Autodesk Fusion 360 part; units mm, degrees
sketch "Sketch1" plane through (0, 0, 0) normal (0, 0, 1) x (1, 0, 0)
  line L0 (0, 0) -> (84.5, 0)
  line L1 (84.5, 0) -> (84.5, 126.75)
  line L2 (84.5, 126.75) -> (0, 126.75)
  line L3 (0, 126.75) -> (0, 0)
  line L4 (0, 126.75) -> (5, 126.75)
  line L5 (5, 126.75) -> (5, 121.75)
  line L6 (5, 121.75) -> (0, 121.75)
  line L7 (0, 121.75) -> (0, 126.75)
  line L8 (84.5, 0) -> (79.5, 0)
  line L9 (79.5, 0) -> (79.5, 5)
  line L10 (79.5, 5) -> (84.5, 5)
  line L11 (84.5, 5) -> (84.5, 0)
  line L12 (5, 121.75) -> (79.5, 121.75)
  line L13 (79.5, 121.75) -> (79.5, 5)
  line L14 (79.5, 5) -> (5, 5)
  line L15 (5, 5) -> (5, 121.75)
  dimension "d1" = 84.5
  dimension "d2" = 126.75
  dimension "d3" = 5
  dimension "d4" = 5
  dimension "d5" = 5
  dimension "d6" = 5
extrude "Extrude1" add sketch "Sketch1" along normal blind 22 contours L0 L3 L6 L9 L14 L15 | L0 L1 L8 L9 L10 L11 | L2 L3 L4 L5 L6 L7 | L1 L2 L5 L10 L12 L13 makes body 1
sketch "Sketch2" plane through (0, 0, 22) normal (0, 0, 1) x (-1, 0, 0)
  line L0 (-79.5, -5) -> (-5, -5)
  line L1 (-5, -5) -> (-5, -121.75)
  line L2 (-5, -121.75) -> (-79.5, -121.75)
  line L3 (-79.5, -121.75) -> (-79.5, -5)
  line L4 (-84.5, -126.75) -> (0, -126.75)
  line L5 (0, -126.75) -> (0, 0)
  line L6 (0, 0) -> (-84.5, 0)
  line L7 (-84.5, 0) -> (-84.5, -126.75)
  line L8 (0, -126.75) -> (7, -126.75)
  line L9 (7, -126.75) -> (7, -133.75)
  line L10 (7, -133.75) -> (0, -133.75)
  line L11 (0, -133.75) -> (0, -126.75)
  line L12 (-84.5, 0) -> (-91.5, 0)
  line L13 (-91.5, 0) -> (-91.5, 7)
  line L14 (-91.5, 7) -> (-84.5, 7)
  line L15 (-84.5, 7) -> (-84.5, 0)
  line L16 (7, -133.75) -> (-91.5, -133.75)
  line L17 (-91.5, -133.75) -> (-91.5, 7)
  line L18 (-91.5, 7) -> (7, 7)
  line L19 (7, 7) -> (7, -133.75)
  line L20 (0, -126.75) -> (0.5, -126.75)
  line L21 (0.5, -126.75) -> (0.5, -127.25)
  line L22 (0.5, -127.25) -> (0, -127.25)
  line L23 (0, -127.25) -> (0, -126.75)
  line L24 (-84.5, 0) -> (-85, 0)
  line L25 (-85, 0) -> (-85, 0.5)
  line L26 (-85, 0.5) -> (-84.5, 0.5)
  line L27 (-84.5, 0.5) -> (-84.5, 0)
  line L28 (0.5, -127.25) -> (-85, -127.25)
  line L29 (-85, -127.25) -> (-85, 0.5)
  line L30 (-85, 0.5) -> (0.5, 0.5)
  line L31 (0.5, 0.5) -> (0.5, -127.25)
  dimension "d9" = 7
  dimension "d10" = 7
  dimension "d11" = 7
  dimension "d12" = 7
  dimension "d24" = 0.5
  dimension "d25" = 0.5
  dimension "d26" = 0.5
  dimension "d27" = 0.5
extrude "Extrude2" add sketch "Sketch2" along normal blind 4 separate body contours L8 L15 L18 L19 L30 L31 | L8 L9 L10 L11 L16 L19 L21 L22 L28 L31 | L11 L12 L16 L17 L28 L29 | L12 L13 L14 L15 L17 L18 L25 L26 L29 L30 makes body 2
chamfer "Chamfer1" distance 2 angle 45 4 edges at (85, 63.375, 26) (42.25, -0.5, 26) (-0.5, 63.375, 26) (42.25, 127.25, 26) on bodies 2
extrude "Extrude3" add sketch "Sketch2" against normal blind 2 contours L4 L7 L11 L12 L23 L24 L28 L29 | L5 L6 L8 L15 L20 L27 L30 L31 | L8 L11 L20 L21 L22 L23 L28 L31 | L12 L15 L24 L25 L26 L27 L29 L30 | L8 L15 L18 L19 L30 L31 | L8 L9 L10 L11 L16 L19 L21 L22 L28 L31 | L11 L12 L16 L17 L28 L29 | L12 L13 L14 L15 L17 L18 L25 L26 L29 L30 bodies 1 2
fillet "Fillet1" radius 2 4 edges at (-7, -7, 24) (91.5, -7, 24) (-7, 133.75, 24) (91.5, 133.75, 24) on bodies 1 2
For this review, take the finished solid that the model builds, in its own axes (mm). A direction names the side the tool comes from. Give positions to 0.01 mm unless a question says otherwise; leave off trailing zeros. Write each loop counter-clockwise with the first axis right and the second up, starting at its lowest first coordinate (ties: lowest second). Pieces come first, ordered by that corner, then holes.
Item 1: Insertion check: P1, Ø4, axis at x = 33.5, z = 15, coming from the -Y side; P2, Ø6, axis at x = 40, z = 10.5, coming from the +Y side; P3, Ø10, axis at y = 43.5, z = 6, coming from the -X side. Each pin has a flat end and moves straight along its axis. Give the tip position at first contact, or say it passes through.
Item 2: Take a section at C-C (z = 7). Give the boundary of the cut face in (x, y).
Item 3: Wall thickness on probe 1 along Y at (x, z) = (49, 23.25); probe 2 along X at (y, z) = (27, 5.25); probe 3 along Y at (x, z) = (35, 16.5): over which ranges is each line inside the solid? List them lowest first.
Item 4: The part is to be moulded in two halves that separate along Y. For faces 1 (the face through (43, 126.75, 10)), 2 (the face through (-7, 62, 23)), 3 (the face through (5, 63, 11)), 4 (the face through (43, -7, 23)), say which applies: +Y half, -Y half, draft (parallel to the pull), parting line (faces both ways), or undercut.
Item 5: Take a section at B-B (y = 7.5). Give the boundary of the cut face in (x, z), and give its area (3 significant figures).
Item 6: Machinability: for faces 5 (the face through (79.5, 64, 11)), 6 (the face through (42, 0, 10)), 7 (the face through (84.5, 62, 10)), 8 (the face through (4, 68, 22)), 9 (the face through (0, 64, 10)), which of the approach directions +Z, -Z, +X, -X, +Y, -Y give a long, thin tool a straight path to every point of the face, cutting with its end or side? Answer none if there is none.
Item 7: Take a section at A-A (x = 45). Give the boundary of the cut face in (y, z).
Established:
1. P1: stops at y = 0
1. P2: stops at y = 126.75
1. P3: stops at x = 0
2. outline: (0, 0) - (84.5, 0) - (84.5, 126.75) - (0, 126.75) - close; hole (5, 5) - (79.5, 5) - (79.5, 121.75) - (5, 121.75) - close
3. probe 1: y = -7 to -0.5, 127.25 to 133.75
3. probe 2: x = 0 to 5, 79.5 to 84.5
3. probe 3: y = 0 to 5, 121.75 to 126.75
4. face 1: +Y half
4. face 2: draft
4. face 3: undercut
4. face 4: -Y half
5. outline: (-7, 20) - (0, 20) - (0, 0) - (5, 0) - (5, 22) - (-0.5, 22) - (-0.5, 24) - (-2.5, 26) - (-7, 26) - close; (79.5, 0) - (84.5, 0) - (84.5, 20) - (91.5, 20) - (91.5, 26) - (87, 26) - (85, 24) - (85, 22) - (79.5, 22) - close
5. area: 296 mm2
6. face 5: +Z, -Z
6. face 6: -Z, +X, -X, -Y
6. face 7: -Z, +X, +Y, -Y
6. face 8: +Z
6. face 9: -Z, -X, +Y, -Y
7. outline: (-7, 20) - (0, 20) - (0, 0) - (5, 0) - (5, 22) - (-0.5, 22) - (-0.5, 24) - (-2.5, 26) - (-7, 26) - close; (121.75, 0) - (126.75, 0) - (126.75, 20) - (133.75, 20) - (133.75, 26) - (129.25, 26) - (127.25, 24) - (127.25, 22) - (121.75, 22) - close
